Work out the finished part from the listing and answer in its coordinate system (mm). A direction names the side the tool comes from. Give positions to 0.01 mm unless a question says otherwise; leave off trailing zeros. Loops run counter-clockwise (first coordinate to the right, second up) from the corner with the lowest first, then second, coordinate; pieces in that order, holes last. Notation, with made-up numbers: M 15,10 L 38,10 A13 cw 38,18 Z; hole C 75,42 d6. An arc over 180 degrees is marked long. Use a Markdown table: item, result.
```python
from build123d import *

# Parameters (mm, degrees)
BOSS_EXTRUDE1_DEPTH = 7.5
SKETCH2_R           = 5
BOSS_EXTRUDE2_DEPTH = 8
SKETCH3_R           = 6.5
CUT_EXTRUDE1_DEPTH  = 13
CUT_EXTRUDE2_REACH  = 25
SKETCH4_R           = 3
CUT_EXTRUDE3_START  = -6.308696
SKETCH5_R           = 4.5
CUT_EXTRUDE3_DEPTH  = 6.308696
SKETCH6_R           = 0.75
CUT_EXTRUDE4_DEPTH  = 2
FILLET1_R           = 1.5


with BuildPart() as part:
    # Sketch1 → Boss-Extrude1 (new body, symmetric)
    with BuildSketch(Plane.XY):
        with BuildLine():
            Line((-12, 0), (12, 0))
            Line((12, 0), (12, 3))
            Line((12, 3), (10, 3))
            ThreePointArc((10, 3), (8.267949192, 4), (8.267949192, 6))
            Line((8.267949192, 6), (11.258330249, 11.179491924))
            Line((11.258330249, 11.179491924), (0, 17.679491924))
            Line((0, 17.679491924), (-11.258330249, 11.179491924))
            Line((-11.258330249, 11.179491924), (-8.267949192, 6))
            ThreePointArc((-8.267949192, 6), (-8.267949192, 4), (-10, 3))
            Line((-10, 3), (-12, 3))
            Line((-12, 3), (-12, 0))
        make_face()
    extrude(amount=BOSS_EXTRUDE1_DEPTH, both=True)

    # Sketch2 → Boss-Extrude2 (add)
    with BuildSketch(Plane.XY.offset(7.5)):
        with Locations(Location((0, 8, 0), (0, 0, 180))):  # turned: the seam where the file's is
            Circle(SKETCH2_R)
    extrude(amount=BOSS_EXTRUDE2_DEPTH)

    # Sketch3 → Cut-Extrude1 (cut)
    with BuildSketch(Plane(origin=(0, 0, -7.5), x_dir=(-1, 0, 0), z_dir=(0, 0, -1))):
        with Locations((0, 8)):
            Circle(SKETCH3_R)
    extrude(amount=-CUT_EXTRUDE1_DEPTH, mode=Mode.SUBTRACT)

    # Sketch4 → Cut-Extrude2 (cut, up to next)
    with BuildSketch(Plane.XY.offset(15.5), mode=Mode.PRIVATE) as cut_extrude2_sk1:
        with Locations((0, 8)):
            Circle(SKETCH4_R)
    cut_extrude2_tool1 = extrude(cut_extrude2_sk1.sketch, amount=-CUT_EXTRUDE2_REACH, mode=Mode.PRIVATE) & part.part
    add(cut_extrude2_tool1.solids().sort_by_distance((0, 8, 15.5))[0], mode=Mode.SUBTRACT)

    # Sketch5 → Cut-Extrude3 (cut)
    with BuildSketch(Plane(origin=(7.655444566, 13.259618943, 0), x_dir=(0.866025404, -0.5, 0), z_dir=(0.5, 0.866025404, 0)).offset(CUT_EXTRUDE3_START)):
        with Locations(Location((-2.339745962, 0, 0), (0, 0, 180))):  # turned: the seam where the file's is
            Circle(SKETCH5_R)
    cut_extrude3 = extrude(amount=CUT_EXTRUDE3_DEPTH, mode=Mode.SUBTRACT)

    # Mirror1: Cut-Extrude3 across plane
    add(cut_extrude3.mirror(Plane(origin=(0, 0, 0), x_dir=(0, 0, 1), z_dir=(1, 0, 0))), mode=Mode.SUBTRACT)

    # Sketch6 → Cut-Extrude4 (cut)
    with BuildSketch(Plane(origin=(7.655444566, 13.259618943, 0), x_dir=(0.866025404, -0.5, 0), z_dir=(0.5, 0.866025404, 0))):
        with Locations(Location((-6.839745962, 4.5, 0), (0, 0, 180))):  # turned: the seam where the file's is
            Circle(SKETCH6_R)
        with Locations(Location((2.160254038, 4.5, 0), (0, 0, 180))):  # turned: the seam where the file's is
            Circle(SKETCH6_R)
        with Locations(Location((2.160254038, -4.5, 0), (0, 0, 180))):  # turned: the seam where the file's is
            Circle(SKETCH6_R)
        with Locations(Location((-6.839745962, -4.5, 0), (0, 0, 180))):  # turned: the seam where the file's is
            Circle(SKETCH6_R)
    cut_extrude4 = extrude(amount=-CUT_EXTRUDE4_DEPTH, mode=Mode.SUBTRACT)

    # Mirror2: Cut-Extrude4 across plane
    add(cut_extrude4.mirror(Plane(origin=(0, 0, 0), x_dir=(0, 0, 1), z_dir=(1, 0, 0))), mode=Mode.SUBTRACT)

    # Fillet1
    fillet1_edges = [part.edges().sort_by_distance(p)[0] for p in [
        (5, 8, 7.5),
    ]]
    fillet(fillet1_edges, radius=FILLET1_R)


solid = part.part
```
(1) Given P1, Ø2, axis at x = -8.5, y = 8, coming from the +Z side; P2, Ø1, axis at y = 4.5, z = 10.5, coming from the -X side; P3, Ø1, axis at x = -4.5, y = 3.5, coming from the +Z side, each flat-ended and moving along its own axis, determine where each tip first touches the part or whether it passes through.
Entries:
| item | result |
|---|---|
| P1 | stops at z = 7.5 |
| P2 | stops at x = -4 |
| P3 | stops at z = 7.64 |
(2) Which of the six approach directions +Z, -Z, +X, -X, +Y, -Y give full straight-line access (tool end or side, diameter ignored) to faces 4 (the flat face through (-3, 7, 5.5)), 5 (the flat face through (8.54, 10.44, 4.51)), 6 (the flat face through (0, 1, -7.5)), 7 (the flat face through (10, 9, 0)), 8 (the flat face through (-11, 3, 0))?
Entries:
| item | result |
|---|---|
| face 4 | -Z |
| face 5 | none |
| face 6 | -Z, +X, -X, +Y, -Y |
| face 7 | +Z, -Z, +X |
| face 8 | +Z, -Z, -X |
(3) A cutting plane is placed at B-B (x = -10.5). Write down the section's boundary in (y, z), and give its area (3 significant figures).
Entries:
| item | result |
|---|---|
| outline | M 0,-7.5 L 3,-7.5 L 3,7.5 L 0,7.5 Z; M 9.87,-7.5 L 11.62,-7.5 L 11.62,7.5 L 9.87,7.5 Z |
| area | 71.3 mm² |
(4) A cutting plane is placed at C-C (z = 12.5). Write down the section's boundary in (x, y).
Entries:
| item | result |
|---|---|
| outline | C 0,8 d10; hole C 0,8 d6 |
(5) The mould has two halves that part along Y. Classify faces 1 (the cylindrical face through (0.651, 3.043, 12.204)), 2 (the flat face through (-3.3, 7.9, 15.5)), 3 (the cylindrical face through (1.38, 15.74, 3.77)): released by +Y, released by -Y, zero draft, split by the parting line, or undercut.
Entries:
| item | result |
|---|---|
| face 1 | split by the parting line |
| face 2 | zero draft |
| face 3 | undercut |
(6) Consider probe 1 along Y at (x, z) = (0, 13.5); probe 2 along Z at (x, y) = (-1, 11); probe 3 along Y at (x, z) = (-10, -6). Determine where each line is inside the solid, lowest interval first. Write a range as [from, to].
Entries:
| item | result |
|---|---|
| probe 1 | y = [3, 5], [11, 13] |
| probe 2 | z = [5.5, 15.5] |
| probe 3 | y = [0, 3], [9, 11.91] |
(7) A cutting plane is placed at D-D (y = 11.5). Count the separate pieces of the cut face and the enclosed holes in it, and give its area (3 significant figures).
Entries:
| item | result |
|---|---|
| separate pieces | 1 |
| enclosed holes | 4 |
| area | 183 mm² |
(8) A cutting plane is placed at A-A (z = 1.25). Write down the section's boundary in (x, y).
Entries:
| item | result |
|---|---|
| outline | M -12,0 L 12,0 L 12,3 L 10,3 A2 cw 8.27,6 L 11.26,11.18 L 9.37,12.27 L 6.45,7.21 A6.5 cw -6.45,7.21 L -9.37,12.27 L -11.26,11.18 L -8.27,6 A2 cw -10,3 L -12,3 Z; M -1.89,16.59 L -0.66,14.47 A6.5 cw 0.66,14.47 L 1.89,16.59 L 0,17.68 Z |
